Autodesk Inventor part; units mm, degrees
ref_plane "YZ Plane" through (0, 0, 0) normal (1, 0, 0) x (0, 1, 0)
ref_plane "XZ Plane" through (0, 0, 0) normal (0, 1, 0) x (-1, 0, 0)
ref_plane "XY Plane" through (0, 0, 0) normal (0, 0, 1) x (1, 0, 0)
sketch "Sketch2" plane through (0, 0, 0) normal (0, 0, 1) x (1, 0, 0)
  circle A0 centre (0, 0) radius 45
  dimension "d0" = 90
extrude "Extrusion1" add sketch "Sketch2" along normal blind 10
sketch "Sketch4" plane through (0, 0, 10) normal (0, 0, 1) x (1, 0, 0)
  circle A0 centre (0, 0) radius 11.5
  dimension "d14" = 23
extrude "Extrusion3" add sketch "Sketch4" along normal blind 23
sketch "Sketch5" plane through (0, 0, 33) normal (0, 0, 1) x (1, 0, 0)
  circle A0 centre (-8, 0) radius 2
  circle A1 centre (0, 0) radius 3.5
  circle A2 centre (0, 0) radius 11.5 construction
  circle A3 centre (-2.4721, -7.6085) radius 2
  circle A4 centre (6.4721, -4.7023) radius 2
  circle A5 centre (6.4721, 4.7023) radius 2
  circle A6 centre (-2.4721, 7.6085) radius 2
  dimension "d19" = 4
  dimension "d20" = 8
  dimension "d21" = 360
  dimension "d22" = 7
extrude "Extrusion4" cut sketch "Sketch5" against normal through all
sketch "Sketch6" plane through (0, 0, 10) normal (0, 0, 1) x (1, 0, 0)
  line L0 (-40, 0) -> (-27.3, 0)
  line L1 (-27.3, 0) -> (-27.3, 12.7)
  line L2 (-27.3, 12.7) -> (-40, 12.7)
  line L3 (-40, 12.7) -> (-40, 0)
  line L4 (-40.5, 13.2) -> (-26.8, 13.2)
  line L5 (-26.8, 13.2) -> (-26.8, -0.5)
  line L6 (-26.8, -0.5) -> (-40.5, -0.5)
  line L7 (-40.5, -0.5) -> (-40.5, 13.2)
  line L8 (-33.6501, -21.6256) -> (-22.9662, -14.7595)
  line L9 (-22.9662, -14.7595) -> (-29.8324, -4.0756)
  line L10 (-29.8324, -4.0756) -> (-40.5163, -10.9417)
  line L11 (-40.5163, -10.9417) -> (-33.6501, -21.6256)
  line L12 (-41.2072, -10.7914) -> (-29.6821, -3.3846)
  line L13 (-29.6821, -3.3846) -> (-22.2753, -14.9098)
  line L14 (-22.2753, -14.9098) -> (-33.8004, -22.3166)
  line L15 (-33.8004, -22.3166) -> (-41.2072, -10.7914)
  line L16 (-16.6166, -36.3853) -> (-11.3408, -24.833)
  line L17 (-11.3408, -24.833) -> (-22.8932, -19.5572)
  line L18 (-22.8932, -19.5572) -> (-28.1689, -31.1095)
  line L19 (-28.1689, -31.1095) -> (-16.6166, -36.3853)
  line L20 (-28.8315, -31.3566) -> (-23.1403, -18.8947)
  line L21 (-23.1403, -18.8947) -> (-10.6783, -24.5858)
  line L22 (-10.6783, -24.5858) -> (-16.3695, -37.0478)
  line L23 (-16.3695, -37.0478) -> (-28.8315, -31.3566)
  line L24 (5.6926, -39.5929) -> (3.8852, -27.0221)
  line L25 (3.8852, -27.0221) -> (-8.6855, -28.8295)
  line L26 (-8.6855, -28.8295) -> (-6.8781, -41.4003)
  line L27 (-6.8781, -41.4003) -> (5.6926, -39.5929)
  line L28 (-7.3019, -41.9663) -> (-9.2516, -28.4058)
  line L29 (-9.2516, -28.4058) -> (4.3089, -26.4561)
  line L30 (4.3089, -26.4561) -> (6.2587, -40.0166)
  line L31 (6.2587, -40.0166) -> (-7.3019, -41.9663)
  line L32 (26.1944, -30.23) -> (17.8777, -20.632)
  line L33 (17.8777, -20.632) -> (8.2797, -28.9487)
  line L34 (8.2797, -28.9487) -> (16.5964, -38.5467)
  line L35 (16.5964, -38.5467) -> (26.1944, -30.23)
  line L36 (16.546, -39.252) -> (7.5744, -28.8983)
  line L37 (7.5744, -28.8983) -> (17.9281, -19.9267)
  line L38 (17.9281, -19.9267) -> (26.8997, -30.2804)
  line L39 (26.8997, -30.2804) -> (16.546, -39.252)
  line L40 (38.3797, -11.2693) -> (26.1942, -7.6913)
  line L41 (26.1942, -7.6913) -> (22.6162, -19.8769)
  line L42 (22.6162, -19.8769) -> (34.8017, -23.4549)
  line L43 (34.8017, -23.4549) -> (38.3797, -11.2693)
  line L44 (35.1406, -24.0755) -> (21.9955, -20.2157)
  line L45 (21.9955, -20.2157) -> (25.8553, -7.0707)
  line L46 (25.8553, -7.0707) -> (39.0003, -10.9304)
  line L47 (39.0003, -10.9304) -> (35.1406, -24.0755)
  line L48 (38.3797, 11.2693) -> (26.1942, 7.6913)
  line L49 (26.1942, 7.6913) -> (29.7722, -4.4943)
  line L50 (29.7722, -4.4943) -> (41.9577, -0.9163)
  line L51 (41.9577, -0.9163) -> (38.3797, 11.2693)
  line L52 (42.5783, -1.2551) -> (29.4333, -5.1149)
  line L53 (29.4333, -5.1149) -> (25.5735, 8.0302)
  line L54 (25.5735, 8.0302) -> (38.7186, 11.8899)
  line L55 (38.7186, 11.8899) -> (42.5783, -1.2551)
  line L56 (26.1944, 30.23) -> (17.8777, 20.632)
  line L57 (17.8777, 20.632) -> (27.4757, 12.3152)
  line L58 (27.4757, 12.3152) -> (35.7924, 21.9133)
  line L59 (35.7924, 21.9133) -> (26.1944, 30.23)
  line L60 (36.4978, 21.9637) -> (27.5262, 11.6099)
  line L61 (27.5262, 11.6099) -> (17.1724, 20.5815)
  line L62 (17.1724, 20.5815) -> (26.144, 30.9353)
  line L63 (26.144, 30.9353) -> (36.4978, 21.9637)
  line L64 (5.6926, 39.5929) -> (3.8852, 27.0221)
  line L65 (3.8852, 27.0221) -> (16.4559, 25.2147)
  line L66 (16.4559, 25.2147) -> (18.2633, 37.7855)
  line L67 (18.2633, 37.7855) -> (5.6926, 39.5929)
  line L68 (18.8294, 38.2092) -> (16.8797, 24.6487)
  line L69 (16.8797, 24.6487) -> (3.3191, 26.5984)
  line L70 (3.3191, 26.5984) -> (5.2688, 40.1589)
  line L71 (5.2688, 40.1589) -> (18.8294, 38.2092)
  line L72 (-16.6166, 36.3853) -> (-11.3408, 24.833)
  line L73 (-11.3408, 24.833) -> (0.2115, 30.1087)
  line L74 (0.2115, 30.1087) -> (-5.0643, 41.6611)
  line L75 (-5.0643, 41.6611) -> (-16.6166, 36.3853)
  line L76 (-4.8172, 42.3236) -> (0.874, 29.8616)
  line L77 (0.874, 29.8616) -> (-11.5879, 24.1704)
  line L78 (-11.5879, 24.1704) -> (-17.2791, 36.6324)
  line L79 (-17.2791, 36.6324) -> (-4.8172, 42.3236)
  line L80 (-33.6501, 21.6256) -> (-22.9662, 14.7595)
  line L81 (-22.9662, 14.7595) -> (-16.1001, 25.4434)
  line L82 (-16.1001, 25.4434) -> (-26.784, 32.3096)
  line L83 (-26.784, 32.3096) -> (-33.6501, 21.6256)
  line L84 (-26.9343, 33.0005) -> (-15.4091, 25.5937)
  line L85 (-15.4091, 25.5937) -> (-22.8159, 14.0685)
  line L86 (-22.8159, 14.0685) -> (-34.3411, 21.4753)
  line L87 (-34.3411, 21.4753) -> (-26.9343, 33.0005)
  point P0 (0, 0)
  dimension "d25" = 12.7
  dimension "d26" = 12.7
  dimension "d27" = 40
  dimension "d28" = 0.5
  dimension "d31" = 360
extrude "Extrusion5" cut sketch "Sketch6" against normal blind 6.35 contours L3 L2 L1 L0 | L4 L5 L6 L7 | L11 L10 L9 L8 | L12 L13 L14 L15 | L19 L18 L17 L16 | L20 L21 L22 L23 | L27 L26 L25 L24 | L28 L29 L30 L31 | L35 L34 L33 L32 | L36 L37 L38 L39 | L43 L42 L41 L40 | L44 L45 L46 L47 | L51 L50 L49 L48 | L52 L53 L54 L55 | L59 L58 L57 L56 | L60 L61 L62 L63 | L67 L66 L65 L64 | L68 L69 L70 L71 | L75 L74 L73 L72 | L76 L77 L78 L79 | L83 L82 L81 L80 | L84 L85 L86 L87
sketch "Sketch8" plane through (0, 0, 33) normal (0, 0, 1) x (1, 0, 0)
  circle A0 centre (2.0086, 6.1819) radius 0.75
  circle A1 centre (-5.2586, 3.8206) radius 0.75
  circle A2 centre (-5.2586, -3.8206) radius 0.75
  circle A3 centre (2.0086, -6.1819) radius 0.75
  circle A4 centre (6.5, 0) radius 0.75
  circle A5 centre (-2.4721, 7.6085) radius 2 construction
  circle A6 centre (6.4721, 4.7023) radius 2 construction
  circle A7 centre (-2.4721, 7.6085) radius 2
  line L0 (6.4721, 4.7023) -> (-2.4721, 7.6085) construction
  line L1 (0, 0) -> (2.0086, 6.1819) construction
  point P0 (2, 6.1554)
  dimension "d44" = 1.5
  dimension "d45" = 6.5
  dimension "d48" = 360
extrude "Extrusion7" cut sketch "Sketch8" against normal through all contours A0 | A1 | A2 | A3 | A4
properties part number "SG02" material "ABS Plastic"
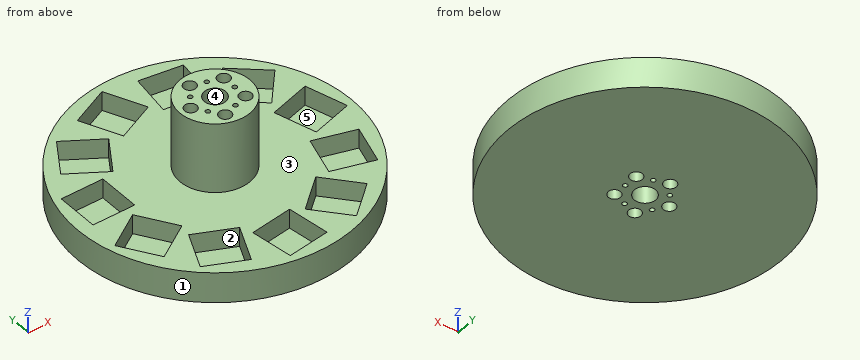
Source: CAD feature listing. Evaluate the final solid. Frame: model axes, mm. Face numbers are marked on the shaded views. A direction names the side the tool comes from. Give positions to 0.01 mm unless a question says otherwise; leave off trailing zeros. Write each loop counter-clockwise with the first axis right and the second up, starting at its lowest first coordinate (ties: lowest second). Pieces come first, ordered by that corner, then holes.
1. Section query A-A (z = 30.5). Count the separate pieces of the cut face and the enclosed holes in it, then the cut area to 3 significant figures.
2. Access query for the marked faces 4 and 5. Directions: +Z, -Z, +X, -X, +Y, -Y. A direction counts if a zero-diameter tool reaches every point of the face in a straight line with its end or side. Return the directions, or none.
3. Material intervals for line 1 along X through (y, z) = (1.5, 26.5); line 2 along Y through (x, z) = (0, 11); line 3 along Y through (x, z) = (6.5, 13.5), sorted ascending.
4. Section query C-C (x = 14.5). Return the cut outline in (y, z), then the cut area to 3 significant figures.
5. Pull-direction query (X, two-part tool) for the marked faces 1, 2 and 3; classes: +X half, -X half, draft (parallel to the pull), parting line (faces both ways), or undercut.
6. Section query B-B (y = 17). Return the cut outline in (x, z).
7. Section query D-D (x = 24). Return the cut outline in (y, z), then the cut area to 3 significant figures.
8. First-contact query: pin 1 (15 mm diameter, centred on x = -31.5, y = 6, fed in from +Z); pin 2 (5 mm diameter, centred on y = -9.5, z = 15, fed in from +X); pin 3 (6 mm diameter, centred on x = -0.5, z = 22, fed in from +Y). Flat tips, straight axial feed; report the tip coordinate or a pass-through.
Output values:
1. separate pieces: 1
1. enclosed holes: 11
1. area: 305 mm2
2. face 4: +Z, -Z
2. face 5: +Z
3. line 1: x = -11.4 to -9.32, -6.68 to -3.16, 3.16 to 11.4
3. line 2: y = -11.5 to -3.5, 3.5 to 11.5
3. line 3: y = -9.49 to -6.7, -2.7 to -0.75, 0.75 to 2.7, 6.7 to 9.49
4. outline: (-42.6, 0) - (42.6, 0) - (42.6, 10) - (38.83, 10) - (38.83, 3.65) - (24.99, 3.65) - (24.99, 10) - (-22.9, 10) - (-22.9, 3.65) - (-36.89, 3.65) - (-36.89, 10) - (-42.6, 10) - close
4. area: 675 mm2
5. face 1: parting line
5. face 2: undercut
5. face 3: draft
6. outline: (-41.67, 0) - (41.67, 0) - (41.67, 10) - (32.2, 10) - (32.2, 3.65) - (21.31, 3.65) - (21.31, 10) - (-20.93, 10) - (-20.93, 3.65) - (-27.38, 3.65) - (-27.38, 10) - (-41.67, 10) - close
7. outline: (-38.07, 0) - (38.07, 0) - (38.07, 10) - (28.46, 10) - (28.46, 3.65) - (14.67, 3.65) - (14.67, 10) - (-13.39, 10) - (-13.39, 3.65) - (-20.8, 3.65) - (-20.8, 10) - (-26.93, 10) - (-26.93, 3.65) - (-32.79, 3.65) - (-32.79, 10) - (-38.07, 10) - close
7. area: 589 mm2
8. pin 1: stops at z = 10
8. pin 2: stops at x = 9.12
8. pin 3: stops at y = 11.5
